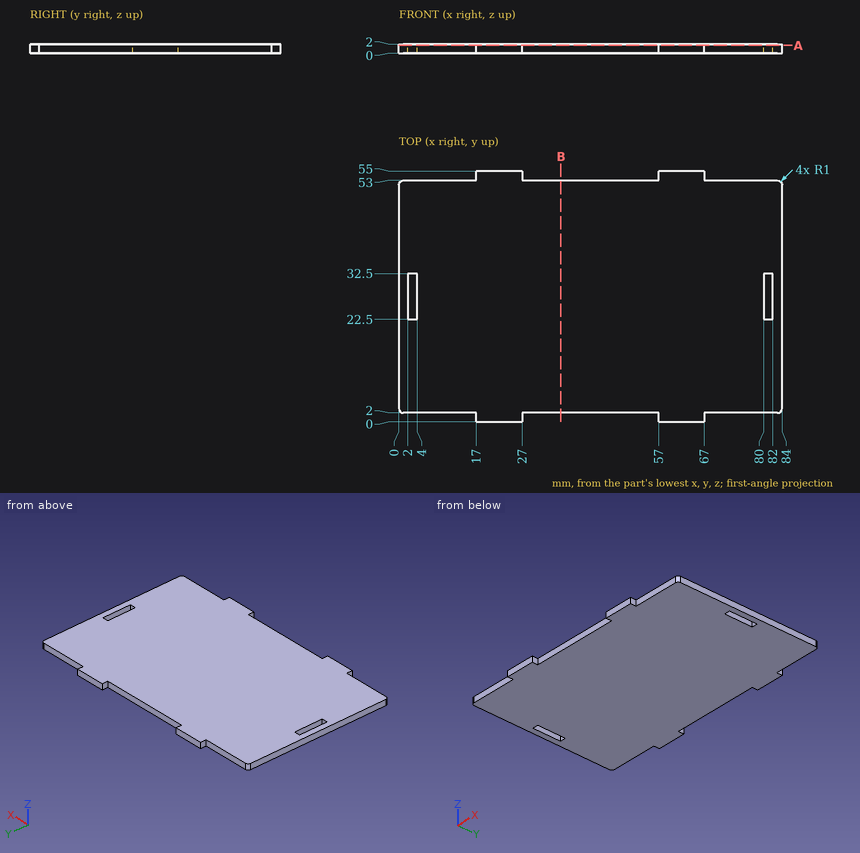
Could you check a few things on this drawing? It's one solid part, dimensions in mm from its lowest x, y, z. Give positions to 0.01 mm unless a question says otherwise; leave off trailing zeros. Write each loop counter-clockwise with the first axis right and the second up, starting at its lowest first coordinate (ties: lowest second). Pieces come first, ordered by that corner, then holes. Notation, with made-up numbers: (-36.75, 62) -> (15.25, 62) arc R15 cw to (15.25, 71) -> close; hole circle Ø6 at (47.5, 79). An arc over 180 degrees is marked (long way). Write each question's results on one line, items separated by ' | '.
1. I want a section at B-B, the plane x = 35.5. Write out the boundary of the cut face in (y, z).
Check sheet entries:
outline: (2, 0) -> (53, 0) -> (53, 2) -> (2, 2) -> close
2. I want a section at A-A, the plane z = 1.7. Count the separate pieces of the cut face and the enclosed holes in it, then the cut area to 3 significant figures.
Check sheet entries:
separate pieces: 1 | enclosed holes: 2 | area: 4,320 mm²
3. I need wall thicknesses on L1, parallel to X at y = 24, z = 0.45; L2, parallel to Y at x = 76, z = 1.05. Which ranges of each line are inside material? Lowest first, please.
Check sheet entries:
L1: x = 0 to 2, 4 to 80, 82 to 84 | L2: y = 2 to 53
4. Will these pins go through, and if not, where does the flat tip stop? pin 1 Ø0.6 at (x, z) = (72.5, 1) entering from -Y; pin 2 Ø0.6 at (x, z) = (74, 0.5) entering from +Y; pin 3 Ø0.6 at (y, z) = (54, 1) entering from +X.
Check sheet entries:
pin 1: stops at y = 2 | pin 2: stops at y = 53 | pin 3: stops at x = 67
